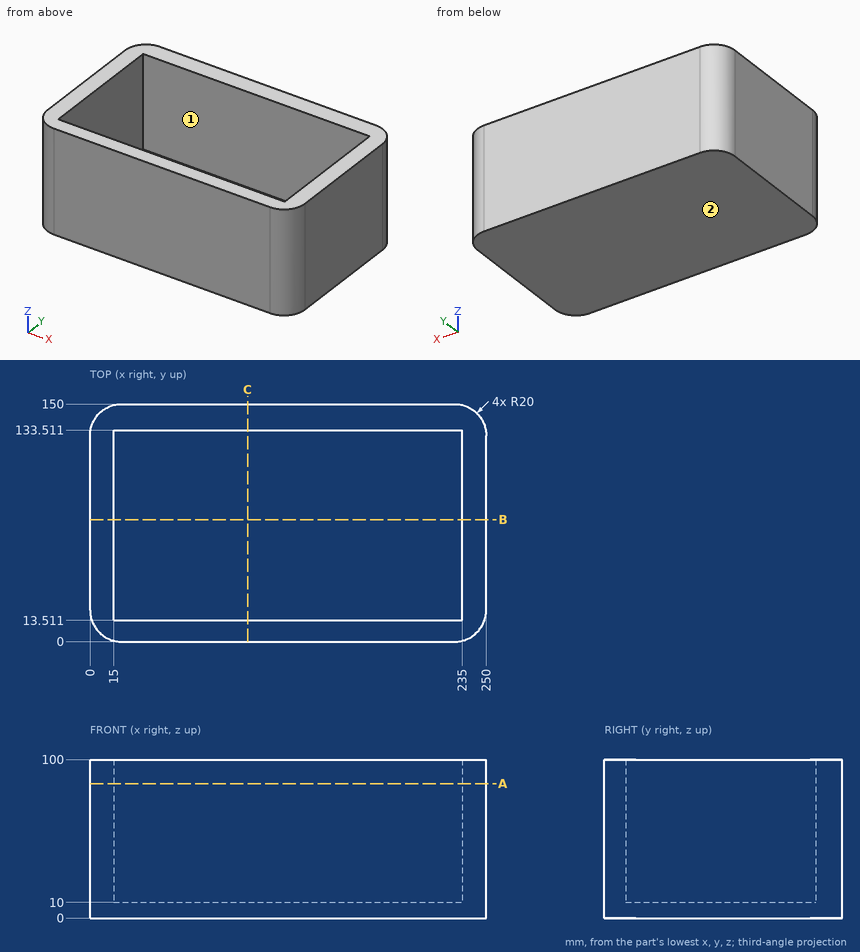
Answer from the drawing. Dimensions are ordinates in mm from the lowest x, y and z of the part. A direction names the side the tool comes from. Give positions to 0.01 mm unless a question says otherwise; leave off trailing zeros. Write each loop counter-clockwise with the first axis right and the second up, starting at its lowest first coordinate (ties: lowest second). Pieces come first, ordered by that corner, then holes. Notation, with made-up numbers: (-3, 39) - (50, 39) arc R14 ccw to (50, 61) - close; hole circle Ø9 at (83.25, 74). An arc over 180 degrees is marked (long way). Answer in a Markdown table with one row per item. Add a question column.
Item 1: Section A-A, the plane z = 85 is taken. Write down the section's boundary in (x, y), and give its area (3 significant figures).
Item 2: A flat-ended cylindrical pin translates along its axis: P1, Ø4, axis at x = 52, y = 97, coming from the +Z side. Find the tip coordinate at first contact, or state that the pin passes through.
Item 3: Find the intervals of material crossed by L1, parallel to X at y = 126.5, z = 59; L2, parallel to Y at x = 186, z = 54.5; L3, parallel to Z at x = 145, y = 120.5, in increasing order.
Item 4: A tool of negligible diameter and unlimited length cuts with its end or side. For the marked faces 1 and 2, from which of +Z, -Z, +X, -X, +Y, -Y can it reach the whole face along a straight path? Write none if from no direction.
Item 5: Section B-B, the plane y = 77 is taken. Write down the section's boundary in (x, z).
Item 6: Section C-C, the plane x = 99.5 is taken. Write down the section's boundary in (y, z), and give its area (3 significant figures).
Recorded:
| question | item | result |
|---|---|---|
| 1 | outline | (0, 20) arc R20 ccw to (20, 0) - (230, 0) arc R20 ccw to (250, 20) - (250, 130) arc R20 ccw to (230, 150) - (20, 150) arc R20 ccw to (0, 130) - close; hole (15, 13.51) - (235, 13.51) - (235, 133.51) - (15, 133.51) - close |
| 1 | area | 10,800 mm2 |
| 2 | P1 | stops at z = 10 |
| 3 | L1 | x = 0 to 15, 235 to 250 |
| 3 | L2 | y = 0 to 13.51, 133.51 to 150 |
| 3 | L3 | z = 0 to 10 |
| 4 | face 1 | +Z |
| 4 | face 2 | -Z, +X, -X, +Y, -Y |
| 5 | outline | (0, 0) - (250, 0) - (250, 100) - (235, 100) - (235, 10) - (15, 10) - (15, 100) - (0, 100) - close |
| 6 | outline | (0, 0) - (150, 0) - (150, 100) - (133.51, 100) - (133.51, 10) - (13.51, 10) - (13.51, 100) - (0, 100) - close |
| 6 | area | 4,200 mm2 |
